```python
from build123d import *

# Parameters (mm, degrees)
F1_DEPTH = 10


# Not quite as in the source:
# - a feature of the source that left no trace in its solid (it failed there, or was rolled back) is left out


with BuildPart() as f1:
    # F0 (on Top) → F1 (new body)
    with BuildSketch(Plane.XY):
        with BuildLine():
            ThreePointArc((5.3398427629, 5.9570193274), (6.9282032303, 4), (7.8288514498, 1.6459298212))
            add(Edge.make_bspline(
                [(7.8288514498, 1.6459298212), (10.3819017266, -1.689149351), (14.3784307752, -4.8466401497), (21.2176223927, -10.25)],
                knots=[22.7730577605, 22.7730577605, 22.7730577605, 22.7730577605, 38.9711431703, 38.9711431703, 38.9711431703, 38.9711431703], degree=3))
            Line((21.2176223927, -10.25), (18.5700532559, -5.6642757385))
            add(Edge.make_bspline(
                [(18.5700532559, -5.6642757385), (8.8931150266, 2.4300062697), (6.5510046742, 6.486660397), (4.3796199444, 18.9142757385)],
                knots=[8.5821930458, 8.5821930458, 8.5821930458, 8.5821930458, 41.6472803737, 41.6472803737, 41.6472803737, 41.6472803737], degree=3))
            Line((4.3796199444, 18.9142757385), (1.7320508076, 23.5))
            add(Edge.make_bspline(
                [(1.7320508076, 23.5), (2.991901895, 14.8754063927), (3.7281046145, 9.8355653103), (5.3398427629, 5.9570193274)],
                knots=[0, 0, 0, 0, 16.1980854098, 16.1980854098, 16.1980854098, 16.1980854098], degree=3))
        make_face()
        with BuildLine():
            add(Edge.make_bspline(
                [(2.4890086869, -7.6029491486), (6.6537971121, -8.1464159593), (11.3865288802, -10.0287662431), (19.4855715851, -13.25)],
                knots=[22.7730577605, 22.7730577605, 22.7730577605, 22.7730577605, 38.9711431703, 38.9711431703, 38.9711431703, 38.9711431703], degree=3))
            ThreePointArc((2.4890086869, -7.6029491486), (0, -8), (-2.4890086869, -7.6029491486))
            add(Edge.make_bspline(
                [(-19.4855715852, -13.25), (-11.3865288802, -10.0287662431), (-6.6537971121, -8.1464159593), (-2.4890086869, -7.6029491486)],
                knots=[0, 0, 0, 0, 16.1980854098, 16.1980854098, 16.1980854098, 16.1980854098], degree=3))
            Line((-19.4855715852, -13.25), (-14.1904333115, -13.25))
            add(Edge.make_bspline(
                [(-14.1904333115, -13.25), (-2.3421103524, -8.9166666667), (2.3421103524, -8.9166666667), (14.1904333115, -13.25)],
                knots=[8.5821930458, 8.5821930458, 8.5821930458, 8.5821930458, 41.6472803737, 41.6472803737, 41.6472803737, 41.6472803737], degree=3))
            Line((14.1904333115, -13.25), (19.4855715851, -13.25))
        make_face()
        with BuildLine():
            Line((18.5700532559, -5.6642757385), (21.2176223927, -10.25))
            ThreePointArc((21.2176223927, -10.25), (21.2176223927, -12.25), (19.4855715851, -13.25))
            Line((19.4855715851, -13.25), (14.1904333115, -13.25))
            add(Edge.make_bspline(
                [(14.1904333115, -13.25), (16.2714670553, -14.0111045817), (18.573507913, -14.9058892059), (21.174191051, -15.9343538726)],
                knots=[41.6472803737, 41.6472803737, 41.6472803737, 41.6472803737, 47.4548164026, 47.4548164026, 47.4548164026, 47.4548164026], degree=3))
            ThreePointArc((21.174191051, -15.9343538726), (22.9496732003, -13.25), (24.386650772, -10.3702104184))
            add(Edge.make_bspline(
                [(24.386650772, -10.3702104184), (22.1956326748, -8.6321850871), (20.2697060304, -7.0859515359), (18.5700532559, -5.6642757385)],
                knots=[2.7746570169, 2.7746570169, 2.7746570169, 2.7746570169, 8.5821930458, 8.5821930458, 8.5821930458, 8.5821930458], degree=3))
        make_face()
        with BuildLine():
            ThreePointArc((-7.8288514498, 1.6459298212), (-6.9282032303, 4), (-5.3398427629, 5.9570193274))
            add(Edge.make_bspline(
                [(-1.7320508076, 23.5), (-2.991901895, 14.8754063927), (-3.7281046145, 9.8355653103), (-5.3398427629, 5.9570193274)],
                knots=[0, 0, 0, 0, 16.1980854098, 16.1980854098, 16.1980854098, 16.1980854098], degree=3))
            Line((-1.7320508076, 23.5), (-4.3796199444, 18.9142757385))
            add(Edge.make_bspline(
                [(-4.3796199444, 18.9142757385), (-6.5510046742, 6.486660397), (-8.8931150266, 2.4300062697), (-18.5700532559, -5.6642757385)],
                knots=[8.5821930458, 8.5821930458, 8.5821930458, 8.5821930458, 41.6472803737, 41.6472803737, 41.6472803737, 41.6472803737], degree=3))
            Line((-18.5700532559, -5.6642757385), (-21.2176223927, -10.25))
            add(Edge.make_bspline(
                [(-7.8288514498, 1.6459298212), (-10.3819017266, -1.689149351), (-14.3784307752, -4.8466401497), (-21.2176223927, -10.25)],
                knots=[22.7730577605, 22.7730577605, 22.7730577605, 22.7730577605, 38.9711431703, 38.9711431703, 38.9711431703, 38.9711431703], degree=3))
        make_face()
        with BuildLine():
            ThreePointArc((-1.7320508076, 23.5), (0, 24.5), (1.7320508076, 23.5))
            Line((1.7320508076, 23.5), (4.3796199444, 18.9142757385))
            add(Edge.make_bspline(
                [(4.3796199444, 18.9142757385), (3.9982389752, 21.0970561175), (3.6221247618, 23.5380742929), (3.2124597211, 26.304564291)],
                knots=[41.6472803737, 41.6472803737, 41.6472803737, 41.6472803737, 47.4548164026, 47.4548164026, 47.4548164026, 47.4548164026], degree=3))
            ThreePointArc((3.2124597211, 26.304564291), (0, 26.5), (-3.2124597211, 26.304564291))
            add(Edge.make_bspline(
                [(-3.2124597211, 26.304564291), (-3.6221247618, 23.5380742929), (-3.9982389752, 21.0970561175), (-4.3796199444, 18.9142757385)],
                knots=[2.7746570169, 2.7746570169, 2.7746570169, 2.7746570169, 8.5821930458, 8.5821930458, 8.5821930458, 8.5821930458], degree=3))
            Line((-4.3796199444, 18.9142757385), (-1.7320508076, 23.5))
        make_face()
        with BuildLine():
            Line((-14.1904333115, -13.25), (-19.4855715852, -13.25))
            ThreePointArc((-19.4855715852, -13.25), (-21.2176223927, -12.25), (-21.2176223927, -10.25))
            Line((-21.2176223927, -10.25), (-18.5700532559, -5.6642757385))
            add(Edge.make_bspline(
                [(-18.5700532559, -5.6642757385), (-20.2697060304, -7.0859515359), (-22.1956326748, -8.6321850871), (-24.386650772, -10.3702104184)],
                knots=[41.6472803737, 41.6472803737, 41.6472803737, 41.6472803737, 47.4548164026, 47.4548164026, 47.4548164026, 47.4548164026], degree=3))
            ThreePointArc((-24.386650772, -10.3702104184), (-22.9496732003, -13.25), (-21.174191051, -15.9343538726))
            add(Edge.make_bspline(
                [(-21.174191051, -15.9343538726), (-18.573507913, -14.9058892059), (-16.2714670553, -14.0111045817), (-14.1904333115, -13.25)],
                knots=[2.7746570169, 2.7746570169, 2.7746570169, 2.7746570169, 8.5821930458, 8.5821930458, 8.5821930458, 8.5821930458], degree=3))
        make_face()
        with BuildLine():
            add(Edge.make_bspline(
                [(27.7128129211, -13), (26.540759526, -12.0747363675), (25.433449915, -11.2005839464), (24.386650772, -10.3702104184)],
                knots=[0, 0, 0, 0, 2.7746570169, 2.7746570169, 2.7746570169, 2.7746570169], degree=3))
            ThreePointArc((24.386650772, -10.3702104184), (22.9496732003, -13.25), (21.174191051, -15.9343538726))
            add(Edge.make_bspline(
                [(21.174191051, -15.9343538726), (22.4167151923, -16.425721759), (23.7274082013, -16.9476038015), (25.1147367097, -17.5)],
                knots=[47.4548164026, 47.4548164026, 47.4548164026, 47.4548164026, 50.2294734195, 50.2294734195, 50.2294734195, 50.2294734195], degree=3))
            ThreePointArc((25.1147367097, -17.5), (27.7128129211, -16), (27.7128129211, -13))
        make_face()
        with BuildLine():
            ThreePointArc((-3.2124597211, 26.304564291), (0, 26.5), (3.2124597211, 26.304564291))
            add(Edge.make_bspline(
                [(3.2124597211, 26.304564291), (3.0167347227, 27.6263057055), (2.8133513247, 29.0223401691), (2.5980762114, 30.5)],
                knots=[47.4548164026, 47.4548164026, 47.4548164026, 47.4548164026, 50.2294734195, 50.2294734195, 50.2294734195, 50.2294734195], degree=3))
            ThreePointArc((2.5980762114, 30.5), (0, 32), (-2.5980762114, 30.5))
            add(Edge.make_bspline(
                [(-2.5980762114, 30.5), (-2.8133513247, 29.0223401691), (-3.0167347227, 27.6263057055), (-3.2124597211, 26.304564291)],
                knots=[0, 0, 0, 0, 2.7746570169, 2.7746570169, 2.7746570169, 2.7746570169], degree=3))
        make_face()
        with BuildLine():
            add(Edge.make_bspline(
                [(-25.1147367097, -17.5), (-23.7274082013, -16.9476038015), (-22.4167151923, -16.425721759), (-21.174191051, -15.9343538726)],
                knots=[0, 0, 0, 0, 2.7746570169, 2.7746570169, 2.7746570169, 2.7746570169], degree=3))
            ThreePointArc((-21.174191051, -15.9343538726), (-22.9496732003, -13.25), (-24.386650772, -10.3702104184))
            add(Edge.make_bspline(
                [(-24.386650772, -10.3702104184), (-25.433449915, -11.2005839464), (-26.540759526, -12.0747363675), (-27.7128129211, -13)],
                knots=[47.4548164026, 47.4548164026, 47.4548164026, 47.4548164026, 50.2294734195, 50.2294734195, 50.2294734195, 50.2294734195], degree=3))
            ThreePointArc((-27.7128129211, -13), (-27.7128129211, -16), (-25.1147367097, -17.5))
        make_face()
    extrude(amount=F1_DEPTH)


solid = f1.part
```
The model under review builds one solid part; all positions refer to its coordinate system, in mm. A direction names the side the tool comes from. Coordinates: 2 decimals unless noted, no trailing zeros. Answer in a Markdown table with one row per item. Add a question column.
Q1. Clearance check with flat-ended pins moving along their axes: pin 1 (2 mm diameter, centred on x = 22.5, z = 6, fed in from -Y); pin 2 (6 mm diameter, centred on y = 26.5, z = 3, fed in from -X); pin 3 (6 mm diameter, centred on y = 2.5, z = 5.5, fed in from -X). State where each tip first meets the part, or that it passes through.
Q2. Draft analysis for pull direction Y (two halves, no side actions). For faces 3 (the face through (-27.735, -15.962, 4.93)), 4 (the face through (0, 24.5, 4.9)), 5 (the face through (0, 32, 5)), state which applies: +Y half, -Y half, draft (parallel to the pull), parting line (faces both ways), or undercut.
Q3. To check wall thickness, follow line 1 along X through (y, z) = (5.5, 4); line 2 along Y through (x, z) = (11, 5.25); line 3 along X through (y, z) = (2, 6.75). State the ranges of each line that lie inside material, in increasing order. Write a range as from..to.
Q4. For faces 1 (the face through (6, 6, 0)), 2 (the face through (6.91, 4.03, 4.93)), list the 3-axis set-ups (+Z, -Z, +X, -X, +Y, -Y) from which the entire face can be reached by the end or side of a thin tool; tool diameter is ignored.
Answers below:
| question | item | result |
|---|---|---|
| 1 | pin 1 | y = -16.86 |
| 1 | pin 2 | x = -3.63 |
| 1 | pin 3 | x = -12.9 |
| 2 | face 3 | parting line |
| 2 | face 4 | undercut |
| 2 | face 5 | +Y half |
| 3 | line 1 | -8.38..-5.81, 5.81..8.38 |
| 3 | line 2 | -12.13..-9.95, -1.8..1.63 |
| 3 | line 3 | -10.7..-7.75, 7.75..10.7 |
| 4 | face 1 | -Z, +X, -X, +Y, -Y |
| 4 | face 2 | +Z, -Z |
